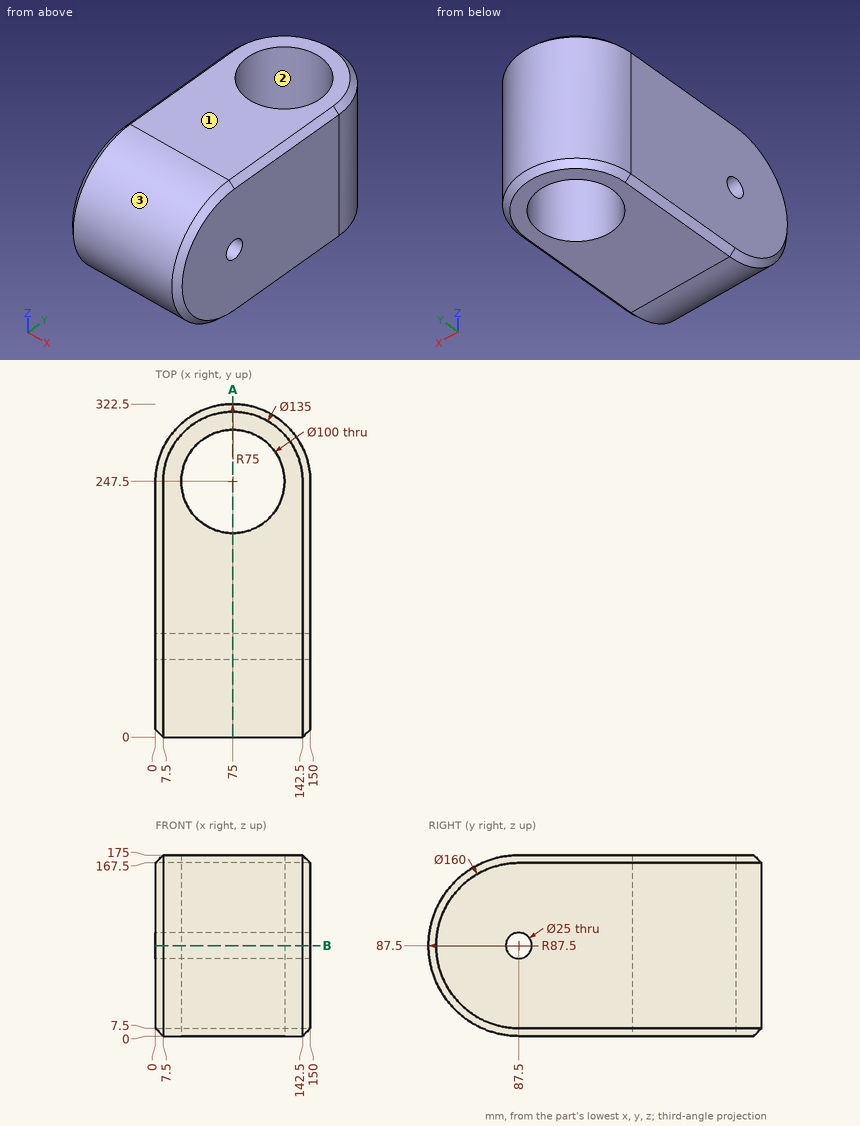
Part print with two shaded views. Sizes in mm from the minimum x, y, z corner. Coordinates: 2 decimals unless noted, no trailing zeros. Order: outer loops, then holes, each group sorted by start corner. A loop starts at its lowest first (then second) coordinate and runs counter-clockwise, first axis right, second up. Notation, with made-up numbers: M 79,-16 L 84,-16 A20 ccw 84,8 Z; hole C 80,-34.75 d8. An arc over 180 degrees is marked long. One line per question, with ' | ' between items. Start each with the question number.
1. Flat gauge pins, fed straight in: P1, Ø1.5, axis at x = 44.5, z = 138.5, coming from the +Y side; P2, Ø5, axis at y = 242, z = 149.5, coming from the -X side; P3, Ø2, axis at y = 274.5, z = 58.5, coming from the -X side; P4, Ø1.5, axis at x = 100.5, y = 46, coming from the +Z side. Where does each tip first touch, or does it go through?
2. Wall check: line 1 along Y through (x, z) = (77, 87.5); line 2 along X through (y, z) = (247, 90); line 3 along Y through (x, z) = (75, 98.5). Give the ranges that are in metal, low to high. Write a range as [from, to].
3. Cut at A-A (x = 75). Write the cut outline in (y, z).
4. Cut at B-B (z = 87.5). Write the cut outline in (x, y), plus the area to 3 significant figures.
5. Mould opens along Y. For the marked faces 1, 2 and 3 say: +Y half, -Y half, draft (parallel to the pull), parting line (faces both ways), or undercut.
The answers:
1) P1: stops at y = 316.35 | P2: stops at x = 0 | P3: stops at x = 4.65 | P4: stops at z = 164.93
2) line 1: y = [0, 75], [100, 197.54], [297.46, 322.47] | line 2: x = [0, 25], [125, 150] | line 3: y = [0.69, 81.56], [93.44, 197.5], [297.5, 322.5]
3) outline: M 87.5,0 L 197.5,0 L 197.5,175 L 87.5,175 A87.5 ccw Z; M 297.5,0 L 315,0 L 322.5,7.5 L 322.5,167.5 L 315,175 L 297.5,175 Z; hole C 87.5,87.5 d25
4) outline: M 0,7.5 L 7.5,0 L 142.5,0 L 150,7.5 L 150,75 L 0,75 Z; M 0,100 L 150,100 L 150,247.5 A75 ccw 0,247.5 Z; hole C 75,247.5 d100 | area: 34,300 mm2
5) face 1: draft | face 2: undercut | face 3: -Y half
